Geometry: see drawing. Coordinates: mm, zero at the bounding-box minimum. A direction names the side the tool comes from. Coordinates: 2 decimals unless noted, no trailing zeros. Loops run counter-clockwise (first coordinate to the right, second up) from the corner with the lowest first, then second, coordinate; pieces in that order, holes last. Notation, with made-up numbers: (87.5, 37) - (106.5, 37) arc R10 ccw to (106.5, 55) - close; hole circle Ø2 at (-2, 10.5). An arc over 180 degrees is marked (long way). Use a Markdown table: item, result. Add a question column.
1. Access query for the marked faces 1, 2, 3 and 4. Directions: +Z, -Z, +X, -X, +Y, -Y. A direction counts if a zero-diameter tool reaches every point of the face in a straight line with its end or side. Return the directions, or none.
2. Section query A-A on y = 20. Return the cut outline in (x, z), then the cut area to 3 significant figures.
3. Section query D-D on z = 3.15. State how many separate pieces and enclosed holes the cut face has, then the cut area to 3 significant figures.
4. Draft query along Y for the marked faces 5, 6, 7 and 8. Return one class per face: released by +Y, released by -Y, zero draft, split by the parting line, or undercut.
5. Section query B-B on x = 17.5. Return the cut outline in (y, z), then the cut area to 4 significant figures.
6. Contact query for flat-ended pins moving along their axis: P1, Ø1.5, axis at x = 4, z = 1.5, coming from the +Y side; P2, Ø1.5, axis at y = 2, z = 3, coming from the +X side; P3, Ø2.5, axis at x = 20.5, z = 2, coming from the +Y side. Output: stop coordinate, or through.
7. Ray query, L1, parallel to Y at x = 9, z = 1.5; L2, parallel to Y at x = 32.5, z = 3.1; L3, parallel to X at y = 37.5, z = 2.7. Return the intervals inside material, ascending. Write a range as [from, to].
8. Section query C-C on y = 2.5. Return the cut outline in (x, z), then the cut area to 3 significant figures.
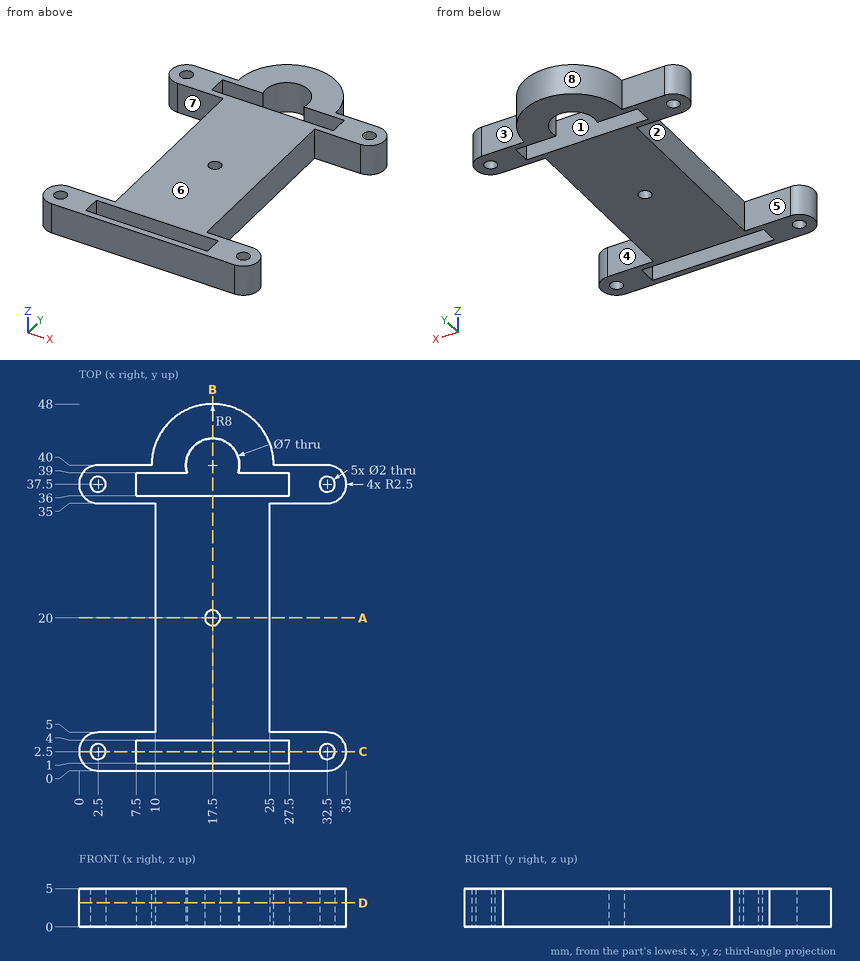
Resolved:
| question | item | result |
|---|---|---|
| 1 | face 1 | +Z, -Z |
| 1 | face 2 | +Z, -Z, -X |
| 1 | face 3 | +Z, -Z, +X, +Y |
| 1 | face 4 | +Z, -Z, +X |
| 2 | outline | (10, 0) - (16.5, 0) - (16.5, 5) - (10, 5) - close; (18.5, 0) - (25, 0) - (25, 5) - (18.5, 5) - close |
| 2 | area | 65.0 mm² |
| 3 | separate pieces | 1 |
| 3 | enclosed holes | 7 |
| 3 | area | 728 mm² |
| 4 | face 5 | undercut |
| 4 | face 6 | zero draft |
| 4 | face 7 | undercut |
| 4 | face 8 | released by +Y |
| 5 | outline | (0, 0) - (1, 0) - (1, 5) - (0, 5) - close; (4, 0) - (19, 0) - (19, 5) - (4, 5) - close; (21, 0) - (36, 0) - (36, 5) - (21, 5) - close; (43.5, 0) - (48, 0) - (48, 5) - (43.5, 5) - close |
| 5 | area | 177.5 mm² |
| 6 | P1 | y = 40 |
| 6 | P2 | x = 35 |
| 6 | P3 | y = 47.81 |
| 7 | L1 | [0, 1], [4, 5], [35, 36], [39, 40] |
| 7 | L2 | [0, 1.5], [3.5, 5], [35, 36.5], [38.5, 40] |
| 7 | L3 | [0, 1.5], [3.5, 7.5], [27.5, 31.5], [33.5, 35] |
| 8 | outline | (0, 0) - (1.5, 0) - (1.5, 5) - (0, 5) - close; (3.5, 0) - (7.5, 0) - (7.5, 5) - (3.5, 5) - close; (27.5, 0) - (31.5, 0) - (31.5, 5) - (27.5, 5) - close; (33.5, 0) - (35, 0) - (35, 5) - (33.5, 5) - close |
| 8 | area | 55.0 mm² |
